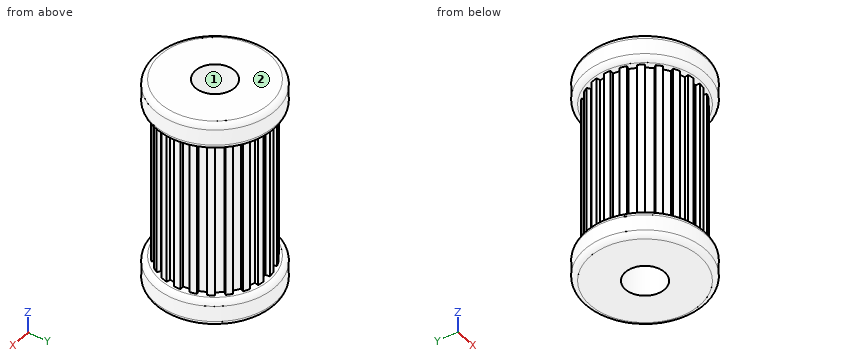
from build123d import *

# Parameters (mm, degrees)
SKETCH1_R           = 20
BOSS_EXTRUDE1_DEPTH = 70
CUT_EXTRUDE1_DEPTH  = 76.498344353
CIRPATTERN1_COUNT   = 22
SKETCH3_R           = 23
BOSS_EXTRUDE2_DEPTH = 10
SKETCH4_R           = 23
BOSS_EXTRUDE3_DEPTH = 10
SKETCH5_R           = 7.5
CUT_EXTRUDE2_DEPTH  = 87.35971283
FILLET1_R           = 2


with BuildPart() as part:
    # Sketch1 → Boss-Extrude1 (new body)
    with BuildSketch(Plane.XY):
        Circle(SKETCH1_R)
    extrude(amount=BOSS_EXTRUDE1_DEPTH)

    # Sketch2 → Cut-Extrude1 (cut, through all)
    with BuildSketch(Plane.XY.offset(70)):
        with BuildLine():
            Line((-1.5, 18.439088915), (1.5, 18.439088915))
            Line((1.5, 18.439088915), (1.621621622, 19.934150178))
            ThreePointArc((1.621621622, 19.934150178), (0, 20), (-1.621621622, 19.934150178))
            Line((-1.621621622, 19.934150178), (-1.5, 18.439088915))
        make_face()
    cut_extrude1 = extrude(amount=-CUT_EXTRUDE1_DEPTH, mode=Mode.SUBTRACT)

    # CirPattern1: Cut-Extrude1 ×22 about axis
    cirpattern1_axis = Axis((0, 0, 0), (0, 0, 1))
    for i in range(1, CIRPATTERN1_COUNT):
        add(cut_extrude1.rotate(cirpattern1_axis, i * 360 / CIRPATTERN1_COUNT), mode=Mode.SUBTRACT)

    # Sketch3 → Boss-Extrude2 (add)
    with BuildSketch(Plane.XY.offset(70)):
        Circle(SKETCH3_R)
    extrude(amount=-BOSS_EXTRUDE2_DEPTH)

    # Sketch4 → Boss-Extrude3 (add)
    with BuildSketch(Plane(origin=(0, 0, 0), x_dir=(-1, 0, 0), z_dir=(0, 0, -1))):
        with Locations(Location((0, 0, 0), (0, 0, 180))):
            Circle(SKETCH4_R)
    extrude(amount=BOSS_EXTRUDE3_DEPTH)

    # Sketch5 → Cut-Extrude2 (cut, through all)
    with BuildSketch(Plane(origin=(0, 0, -10), x_dir=(-1, 0, 0), z_dir=(0, 0, -1))):
        Circle(SKETCH5_R)
    extrude(amount=-CUT_EXTRUDE2_DEPTH, mode=Mode.SUBTRACT)

    # Fillet1
    fillet1_edges = [part.edges().sort_by_distance(p)[0] for p in [
        (-23, 0, 70),
        (-23, 0, 60),
        (-23, 0, 0),
        (-23, 0, -10),
    ]]
    fillet(fillet1_edges, radius=FILLET1_R)


solid = part.part
Can you work these out from the model? Positions are in its coordinate system, mm. Face numbers are marked on the shaded views. Give positions to 0.01 mm unless a question says otherwise; leave off trailing zeros. Order: outer loops, then holes, each group sorted by start corner. A loop starts at its lowest first (then second) coordinate and runs counter-clockwise, first axis right, second up. Notation, with made-up numbers: M 33.25,23.25 L 71.25,23.25 A9 ccw 71.25,27.25 Z; hole C 5.5,-21.5 d11. An arc over 180 degrees is marked long. Use a Markdown table: item, result. Add a question column.
Item 1: Suppose I cut it at B-B (y = 0). List the corners of the cut face in (x, z) for me.
Item 2: We'd pull the mould along Y, two halves only. Please class the marked faces 1 and 2: +Y half, -Y half, draft (parallel to the pull), parting line (faces both ways), or undercut.
Item 3: If I drill on L1, parallel to Y at x = 0.5, z = 37; L2, parallel to X at y = -15, z = 17; L3, parallel to Z at x = -7, y = -18.5, over which ranges is the centre line in solid material (lowest first)? Write a range as [from, to].
Item 4: Suppose I cut it at A-A (x = 0). List the corners of the cut face in (y, z) for me, then the cut area to 3 significant figures.
Item 5: Will these pins go through, and if not, where does the flat tip stop? pin 1 (4 mm diameter, centred on x = -6.5, z = 11.5, fed in from -Y); pin 2 (0.9 mm diameter, centred on x = 0, z = 25.5, fed in from -Y); pin 3 (10 mm diameter, centred on x = -7, z = 15, fed in from -Y); pin 4 (12 mm diameter, centred on x = 0, y = 0, fed in from +Z).
Answer sheet:
| question | item | result |
|---|---|---|
| 1 | outline | M -23,-8 A2 ccw -21,-10 L -7.5,-10 L -7.5,70 L -21,70 A2 ccw -23,68 L -23,62 A2 ccw -21,60 L -20,60 L -20,0 L -21,0 A2 ccw -23,-2 Z; M 7.5,-10 L 21,-10 A2 ccw 23,-8 L 23,-2 A2 ccw 21,0 L 20,0 L 20,60 L 21,60 A2 ccw 23,62 L 23,68 A2 ccw 21,70 L 7.5,70 Z |
| 2 | face 1 | undercut |
| 2 | face 2 | draft |
| 3 | L1 | y = [-18.44, -7.48], [7.48, 18.44] |
| 3 | L2 | x = [-13.23, -11.46], [-10.77, 10.77], [11.46, 13.23] |
| 3 | L3 | z = [-10, 0], [60, 70] |
| 4 | outline | M -23,-8 A2 ccw -21,-10 L -7.5,-10 L -7.5,70 L -21,70 A2 ccw -23,68 L -23,62 A2 ccw -21,60 L -18.44,60 L -18.44,0 L -21,0 A2 ccw -23,-2 Z; M 7.5,-10 L 21,-10 A2 ccw 23,-8 L 23,-2 A2 ccw 21,0 L 18.44,0 L 18.44,60 L 21,60 A2 ccw 23,62 L 23,68 A2 ccw 21,70 L 7.5,70 Z |
| 4 | area | 1,930 mm² |
| 5 | pin 1 | stops at y = -18.67 |
| 5 | pin 2 | stops at y = -18.44 |
| 5 | pin 3 | stops at y = -19.9 |
| 5 | pin 4 | passes through |
